Here's how the part is built. I have some questions about the finished solid (model axes, mm). Face numbers are marked on the shaded views. A direction names the side the tool comes from. Round coordinates to 2 decimals unless told otherwise and drop trailing zeros. Write each loop counter-clockwise with the first axis right and the second up, starting at its lowest first coordinate (ties: lowest second). Pieces come first, ordered by that corner, then holes. Notation, with made-up numbers: (-27.5, 30) -> (-16.5, 30) arc R29 ccw to (-16.5, 65) -> close; hole circle Ø2 at (-31, -29.5). An arc over 180 degrees is marked (long way). Put each result on its own line as item: value. Start each with the question number.
1. We'd pull the mould along X, two halves only. Please class the marked faces 3, 4 and 5: +X half, -X half, draft (parallel to the pull), parting line (faces both ways), or undercut.
2. Suppose I cut it at A-A (y = 7.25). Please give me the cut outline in (x, z) (3 decimals), then the cut area to 3 significant figures.
3. Which directions (+Z, -Z, +X, -X, +Y, -Y) give clear straight access to the entire face, cutting with the end or side of a thin tool? Please do the marked faces 1 and 2.
4. For pin 1 (1 mm diameter, centred on x = 0, z = 0.5, fed in from -Y); pin 2 (1.5 mm diameter, centred on x = 1, y = 4.5, fed in from +Z); pin 3 (3 mm diameter, centred on x = 7.5, y = 3, fed in from +Z); pin 4 (4 mm diameter, centred on x = -0.5, y = 5.5, fed in from -Z), each with a flat end and sliding along its axis, tell me the tip position at first contact or that it passes through.
5. Suppose I cut it at B-B (z = 0). Please give me the cut outline in (x, y).
6. I need wall thicknesses on probe 1 along Y at (x, z) = (-2, 6); probe 2 along Z at (x, y) = (-1, 5.25) (3 decimals); probe 3 along X at (y, z) = (2, -4.5). Which ranges of each line are inside material? Lowest first, please. Write a range as from..to.
7. Suppose I cut it at D-D (z = 2.5). Please give me the cut outline in (x, y).
8. Suppose I cut it at C-C (x = 0). Please give me the cut outline in (y, z) (3 decimals), then the cut area to 3 significant figures.
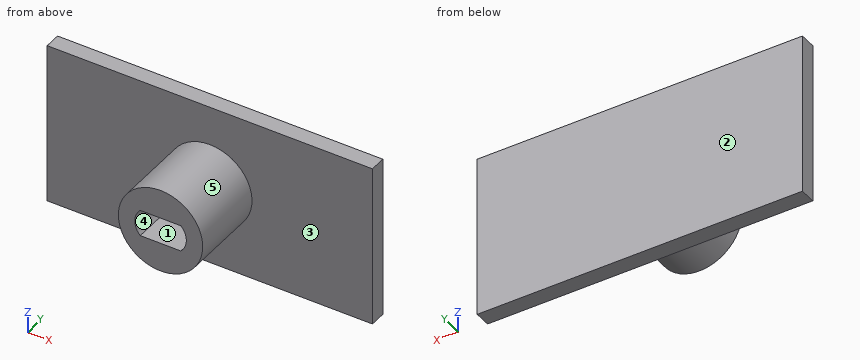
```python
from build123d import *

# Parameters (mm, degrees)
SKETCH2_R           = 5.189332
BOSS_EXTRUDE1_DEPTH = 9.5
CUT_EXTRUDE1_DEPTH  = 11.8
SKETCH5_W           = 40
SKETCH5_H           = 20
BOSS_EXTRUDE2_DEPTH = 2


with BuildPart() as part:
    # Sketch2 → Boss-Extrude1 (new body)
    with BuildSketch(Plane(origin=(0, 0, 0), x_dir=(1, 0, 0), z_dir=(0, 1, 0))):
        with Locations(Location((0, 0, 0), (0, 0, 270))):
            Circle(SKETCH2_R)
    extrude(amount=BOSS_EXTRUDE1_DEPTH)

    # Sketch4 → Cut-Extrude1 (cut)
    with BuildSketch(Plane(origin=(0, 9.5, 0), x_dir=(1, 0, 0), z_dir=(0, 1, 0))):
        with BuildLine():
            Line((0, 1.625), (-2.5, 1.625))
            ThreePointArc((-2.5, 1.625), (-3.173097039, 0), (-2.5, -1.625))
            Line((-2.5, -1.625), (0, -1.625))
            Line((0, -1.625), (0, 0))
            Line((0, 0), (0, 1.625))
        make_face()
        with BuildLine():
            ThreePointArc((2.5, 1.625), (3.173097039, 0), (2.5, -1.625))
            Line((2.5, -1.625), (0, -1.625))
            Line((0, -1.625), (0, 0))
            Line((0, 0), (0, 1.625))
            Line((0, 1.625), (2.5, 1.625))
        make_face()
    extrude(amount=-CUT_EXTRUDE1_DEPTH, mode=Mode.SUBTRACT)

    # Sketch5 → Boss-Extrude2 (add)
    with BuildSketch(Plane(origin=(0, 9.5, 0), x_dir=(1, 0, 0), z_dir=(0, 1, 0))):
        Rectangle(SKETCH5_W, SKETCH5_H)
    extrude(amount=BOSS_EXTRUDE2_DEPTH)


solid = part.part
```
Verdict:
1. face 3: draft
1. face 4: undercut
1. face 5: parting line
2. outline: circle Ø10.379 at (0, 0); hole (-2.5, -1.625) -> (2.5, -1.625) arc R2.298 ccw to (2.5, 1.625) -> (-2.5, 1.625) arc R2.298 ccw to start
2. area: 65.3 mm^2
3. face 1: -Y
3. face 2: +Z, -Z, +X, -X, +Y
4. pin 1: stops at y = 9.5
4. pin 2: stops at z = 5.18
4. pin 3: passes through
4. pin 4: stops at z = -5.19
5. outline: (-20, 9.5) -> (-5.19, 9.5) -> (-5.19, 0) -> (-3.17, 0) -> (-3.17, 9.5) -> (3.17, 9.5) -> (3.17, 0) -> (5.19, 0) -> (5.19, 9.5) -> (20, 9.5) -> (20, 11.5) -> (-20, 11.5) -> close
6. probe 1: y = 9.5..11.5
6. probe 2: z = -5.092..-1.625, 1.625..5.092
6. probe 3: x = -2.58..2.58
7. outline: (-20, 9.5) -> (-4.55, 9.5) -> (-4.55, 0) -> (4.55, 0) -> (4.55, 9.5) -> (20, 9.5) -> (20, 11.5) -> (-20, 11.5) -> close
8. outline: (0, -5.189) -> (9.5, -5.189) -> (9.5, -10) -> (11.5, -10) -> (11.5, 10) -> (9.5, 10) -> (9.5, 5.189) -> (0, 5.189) -> (0, 1.625) -> (9.5, 1.625) -> (9.5, -1.625) -> (0, -1.625) -> close
8. area: 108 mm^2
